Read the model definition and answer for the solid it produces. Units are mm, in the model's axes. A direction names the side the tool comes from. Round coordinates to 2 decimals unless told otherwise and drop trailing zeros. Order: outer loops, then holes, each group sorted by start corner. A loop starts at its lowest first (then second) coordinate and runs counter-clockwise, first axis right, second up. Notation, with made-up numbers: (34, 77) -> (66, 77) arc R15 cw to (66, 90) -> close; hole circle Ø6 at (-2.75, 57.25). An arc over 180 degrees is marked (long way). Use a Markdown table: item, result. Add a question column.
1. The mould has two halves that part along Z. Classify faces 5 (the face through (-13.524, 0.837, 12.288)), 6 (the face through (-8, 14.75, -22)), 7 (the face through (-8, 7, -48.412)), 8 (the face through (0, 3, 43.6)): +Z half, -Z half, draft (parallel to the pull), parting line (faces both ways), or undercut.
2. Section C-C, the plane x = -2 is taken. Give the vertices of the cut face in (y, z), then the cut area to 3 significant figures.
3. Given pin 1 (1.7 mm diameter, centred on x = -12.125, z = 46.35, fed in from -Y) (1 decimal); pin 2 (2 mm diameter, centred on x = -6.5, y = 6.5, fed in from -Z); pin 3 (1 mm diameter, centred on x = 4, y = 6, fed in from +Z); pin 4 (19 mm diameter, centred on x = -10.5, z = -19, fed in from +Y), each flat-ended and moving along its own axis, determine where each tip first touches the part or whether it passes through.
4. For faces 1 (the face through (-3.5, 3, 46)), 2 (the face through (3.5, 3, 46)), 3 (the face through (-8, 12.25, -45)), 4 (the face through (-3.825, 17, -37)), determine the directions among +Z, -Z, +X, -X, +Y, -Y from which every point of the face is accessible in a straight line to the end or side of a thin tool.
5. Section D-D, the plane z = -15.5 is taken. Give the vertices of the cut face in (x, y) (3 decimals).
6. Consider L1, parallel to X at y = 0.7, z = 46.35 (3 decimals); L2, parallel to Z at x = -6.5, y = 8.25; L3, parallel to Z at x = 10.5, y = 6.5. Determine where each line is inside the solid, lowest interval first. Write a range as [from, to].
7. Section B-B, the plane z = 46.35 is taken. Give the vertices of the cut face in (x, y) (3 decimals), then the cut area to 3 significant figures.
8. Section A-A, the plane y = 2.75 is taken. Give the vertices of the cut face in (x, z) (3 decimals).
Autodesk Inventor part; units mm, degrees
ref_plane "YZ Plane" through (0, 0, 0) normal (1, 0, 0) x (0, 1, 0)
ref_plane "XZ Plane" through (0, 0, 0) normal (0, 1, 0) x (-1, 0, 0)
ref_plane "XY Plane" through (0, 0, 0) normal (0, 0, 1) x (1, 0, 0)
sketch "Sketch1" plane through (0, 0, 0) normal (0, 1, 0) x (-1, 0, 0)
  line L0 (16.375, 48.6) -> (-16.375, 48.6)
  line L1 (-16.375, 48.6) -> (-16.375, -48.6)
  line L2 (-16.375, -48.6) -> (16.375, -48.6)
  line L3 (16.375, -48.6) -> (16.375, 48.6)
  line L4 (16.375, 48.6) -> (-16.375, -48.6) construction
  line L5 (-16.375, 48.6) -> (16.375, -48.6) construction
  point P0 (0, 0)
  dimension "d0" = 32.75
  dimension "d1" = 97.2
extrude "Extrusion1" add sketch "Sketch1" along normal blind 1.65
sketch "Sketch3" plane through (0, 1.65, 0) normal (0, 1, 0) x (1, 0, 0)
  line L0 (-16.375, 48.6) -> (-16.375, -48.6)
  line L1 (-16.375, 41.6) -> (1.125, 41.6)
  line L2 (1.125, 41.6) -> (1.125, 1.1)
  line L3 (1.125, 1.1) -> (-16.375, 1.1)
  line L4 (-16.375, 1.1) -> (-16.375, 41.6)
  line L5 (16.375, 48.6) -> (-16.375, 48.6)
  point P0 (0, 0)
  dimension "d7" = 17.5
  dimension "d8" = 40.5
  dimension "d9" = 7
extrude "Extrusion3" add sketch "Sketch3" along normal blind 13.1
sketch "Sketch4" plane through (0, 1.65, 0) normal (0, 1, 0) x (1, 0, 0)
  line L0 (-16.375, 41.6) -> (1.125, 41.6)
  line L1 (-4.075, 41.6) -> (-11.075, 41.6)
  line L2 (-11.075, 41.6) -> (-11.075, 48.4118)
  line L3 (-11.075, 48.4118) -> (-4.075, 48.4118)
  line L4 (-4.075, 48.4118) -> (-4.075, 41.6)
  line L5 (-16.375, 48.6) -> (-16.375, 41.6)
  point P0 (0, 0)
  dimension "d12" = 7
  dimension "d13" = 5.3
extrude "Extrusion4" add sketch "Sketch4" along normal blind 10.6
sketch "Sketch5" plane through (0, 14.75, 0) normal (0, 1, 0) x (1, 0, 0)
  line L0 (1.125, 41.6) -> (-16.375, 41.6)
  line L1 (-16.375, 41.6) -> (-16.375, 1.1)
  line L2 (-16.375, 1.1) -> (1.125, 1.1)
  line L3 (1.125, 1.1) -> (1.125, 41.6)
  line L4 (-11.075, 48.4118) -> (-11.075, 41.6)
  line L5 (-4.075, 41.6) -> (-11.075, 41.6)
  line L6 (-4.075, 41.6) -> (-4.075, 48.4118)
  line L7 (-4.075, 48.4118) -> (-11.075, 48.4118)
  line L8 (-4.075, 41.6) -> (-11.075, 41.6)
  line L9 (-3.825, 41.6) -> (-11.325, 41.6)
  line L10 (-11.325, 41.6) -> (-11.325, 32.3)
  line L11 (-11.325, 32.3) -> (-3.825, 32.3)
  line L12 (-3.825, 32.3) -> (-3.825, 41.6)
  point P0 (0, 0)
  point P1 (-7.575, 41.6)
  dimension "d16" = 9.3
  dimension "d17" = 7.5
extrude "Extrusion5" add sketch "Sketch5" along normal blind 4.46 contours L12 L11 L10 L0
sketch "Sketch6" plane through (-4.075, 1.65, -48.4118) normal (0, 0, -1) x (-1, 0, 0)
  point P0 (-4.075, -1.65)
sketch "Sketch7" plane through (0, 1.65, 0) normal (0, 1, 0) x (1, 0, 0)
  line L0 (-11.325, 32.3) -> (-11.325, 41.6)
  line L1 (-11.325, 41.6) -> (-16.375, 41.6)
  line L2 (-16.375, 41.6) -> (-16.375, 1.1)
  line L3 (-16.375, 1.1) -> (1.125, 1.1)
  line L4 (1.125, 1.1) -> (1.125, 41.6)
  line L5 (1.125, 41.6) -> (-3.825, 41.6)
  line L6 (-3.825, 41.6) -> (-3.825, 32.3)
  line L7 (-3.825, 32.3) -> (-11.325, 32.3)
  line L8 (16.375, -48.6) -> (16.375, 48.6)
  line L9 (-16.375, 48.6) -> (-16.375, -48.6)
  line L10 (16.375, -2.3) -> (-16.375, -2.3)
  line L11 (-16.375, -2.3) -> (-16.375, -4.9)
  line L12 (-16.375, -4.9) -> (16.375, -4.9)
  line L13 (16.375, -4.9) -> (16.375, -2.3)
  point P0 (0, 0)
  point P1 (-16.375, -2.3)
  dimension "d20" = 2.6
  dimension "d21" = 3.4
extrude "Extrusion6" add sketch "Sketch7" along normal blind 8.65 contours L10 L8 L12 L9
sketch "Sketch8" plane through (0, 1.65, 0) normal (0, 1, 0) x (1, 0, 0)
  circle A0 centre (-12.125, -46.35) radius 1.4
  line L0 (-16.375, -4.9) -> (-16.375, -48.6)
  line L1 (-16.375, -48.6) -> (16.375, -48.6)
  circle A1 centre (-12.125, -12.35) radius 1.4
  line L2 (0, -48.6) -> (0, 0) construction
  circle A2 centre (12.125, -46.35) radius 1.4
  circle A3 centre (12.125, -12.35) radius 1.4
  dimension "d24" = 2.8
  dimension "d25" = 4.25
  dimension "d26" = 2.25
  dimension "d27" = 34
extrude "Extrusion7" cut sketch "Sketch8" against normal up to surface (1.65 mm away)
sketch "Sketch9" plane through (0, 1.65, 0) normal (0, 1, 0) x (1, 0, 0)
  line L0 (-16.375, -48.6) -> (16.375, -48.6)
  line L1 (3.5, -43.6) -> (-3.5, -43.6)
  line L2 (-3.5, -43.6) -> (-3.5, -48.6)
  line L3 (-3.5, -48.6) -> (3.5, -48.6)
  line L4 (3.5, -48.6) -> (3.5, -43.6)
  line L5 (3.5, -43.6) -> (-3.5, -48.6) construction
  line L6 (-3.5, -43.6) -> (3.5, -48.6) construction
  point P0 (0, 0)
  point P1 (0, -46.1)
  point P2 (0, -48.6)
  dimension "d30" = 5
  dimension "d31" = 7
extrude "Extrusion8" add sketch "Sketch9" along normal blind 3
properties part number "PCB Board"
Verdict:
| question | item | result |
|---|---|---|
| 1 | face 5 | undercut |
| 1 | face 6 | draft |
| 1 | face 7 | -Z half |
| 1 | face 8 | undercut |
| 2 | outline | (0, -48.6) -> (1.65, -48.6) -> (1.65, -41.6) -> (14.75, -41.6) -> (14.75, -1.1) -> (1.65, -1.1) -> (1.65, 2.3) -> (10.3, 2.3) -> (10.3, 4.9) -> (1.65, 4.9) -> (1.65, 43.6) -> (4.65, 43.6) -> (4.65, 48.6) -> (0, 48.6) -> close |
| 2 | area | 728 mm2 |
| 3 | pin 1 | passes through |
| 3 | pin 2 | stops at z = -48.41 |
| 3 | pin 3 | stops at z = 4.9 |
| 3 | pin 4 | stops at y = 14.75 |
| 4 | face 1 | +Z, -X, +Y |
| 4 | face 2 | +Z, +X, +Y |
| 4 | face 3 | -Z, +X, -X, +Y |
| 4 | face 4 | +Z, -Z, +X, +Y |
| 5 | outline | (-16.375, 0) -> (16.375, 0) -> (16.375, 1.65) -> (1.125, 1.65) -> (1.125, 14.75) -> (-16.375, 14.75) -> close |
| 6 | L1 | x = [-16.375, -13.525], [-10.725, 10.725], [13.525, 16.375] |
| 6 | L2 | z = [-48.41, -1.1], [2.3, 4.9] |
| 6 | L3 | z = [2.3, 4.9] |
| 7 | outline | (-16.375, 0) -> (-13.525, 0) -> (-13.525, 1.65) -> (-16.375, 1.65) -> close; (-10.725, 0) -> (10.725, 0) -> (10.725, 1.65) -> (3.5, 1.65) -> (3.5, 4.65) -> (-3.5, 4.65) -> (-3.5, 1.65) -> (-10.725, 1.65) -> close; (13.525, 0) -> (16.375, 0) -> (16.375, 1.65) -> (13.525, 1.65) -> close |
| 7 | area | 65.8 mm2 |
| 8 | outline | (-16.375, -41.6) -> (-11.075, -41.6) -> (-11.075, -48.412) -> (-4.075, -48.412) -> (-4.075, -41.6) -> (1.125, -41.6) -> (1.125, -1.1) -> (-16.375, -1.1) -> close; (-16.375, 2.3) -> (16.375, 2.3) -> (16.375, 4.9) -> (-16.375, 4.9) -> close; (-3.5, 43.6) -> (3.5, 43.6) -> (3.5, 48.6) -> (-3.5, 48.6) -> close |
